Input: part model. Units: mm. Frame: model coordinates. Coordinates: 2 decimals unless noted, no trailing zeros. Write each loop counter-clockwise with the first axis right and the second up, starting at its lowest first coordinate (ties: lowest second). Pieces come first, ordered by that corner, then holes. Notation, with made-up numbers: (-18.75, 47.5) -> (11.25, 47.5) arc R34 cw to (11.25, 81.5) -> close; hole circle Ø4 at (-16.5, 6). An arc over 180 degrees is marked (long way). Use one line per item in the form item = value. Start each with the question number.
(1) Ray query, line 1 along Z through (x, y) = (-4.5, 0); line 2 along Y through (x, z) = (-4.4, 290); line 3 along Y through (x, z) = (-1, 153.5). Return the intervals inside material, ascending.
(2) Cut plane C-C on z = 158. Return the cut outline in (x, y).
(3) First-contact query: pin 1 (1.5 mm diameter, centred on x = 2, y = 0.5, fed in from -Z). Flat tip, straight axial feed; report the tip coordinate or a pass-through.
(4) Cut plane A-A on x = 0. Return the cut outline in (y, z), plus the area to 3 significant figures.
(5) Cut plane B-B on y = 0. Return the cut outline in (x, z).
Autodesk Inventor part; units mm, degrees
ref_plane "YZ Plane" through (0, 0, 0) normal (1, 0, 0) x (0, 1, 0)
ref_plane "XZ Plane" through (0, 0, 0) normal (0, 1, 0) x (-1, 0, 0)
ref_plane "XY Plane" through (0, 0, 0) normal (0, 0, 1) x (1, 0, 0)
sketch "スケッチ1" plane through (0, 0, 0) normal (0, 0, 1) x (1, 0, 0)
  line L0 (5, -5) -> (-5, -5)
  line L1 (-5, -5) -> (-5, 5)
  line L2 (-5, 5) -> (5, 5)
  line L3 (5, 5) -> (5, -5)
  line L4 (5, -5) -> (-5, 5) construction
  line L5 (-5, -5) -> (5, 5) construction
  line L6 (4, 4) -> (-4, 4)
  line L7 (-4, 4) -> (-4, -4)
  line L8 (-4, -4) -> (4, -4)
  line L9 (4, -4) -> (4, 4)
  point P0 (0, 0)
  dimension "d0" = 10
  dimension "d1" = 10
  dimension "d2" = 1
extrude "押し出し1" add sketch "スケッチ1" along normal blind 300
sketch "スケッチ2" plane through (5, -5, 0) normal (1, 0, 0) x (0, 0, -1)
  line L0 (0, 0) -> (0, 10)
  line L1 (0, 10) -> (-300, 10)
  line L2 (-300, 0) -> (-300, 10)
  line L3 (0, 0) -> (-300, 0)
  line L4 (-300, 5) -> (0, 5)
  point P0 (-290, 5)
  point P1 (-10, 5)
  dimension "d5" = 280
  dimension "d7" = 10
hole "穴1" at (5, 0, 290) at (5, 0, 10) direction (-1, 0, 0) diameter 3.3 end through all
sketch "スケッチ3" plane through (-5, 5, 0) normal (0, 1, 0) x (1, 0, 0)
  line L0 (10, 0) -> (0, 0)
  line L1 (0, 0) -> (0, -300)
  line L2 (10, -300) -> (0, -300)
  line L3 (10, 0) -> (10, -300)
  line L4 (5, 0) -> (5, -300)
  point P0 (5, -150)
hole "穴2" at (0, 5, 150) direction (0, -1, 0) diameter 3.3 end through all
properties part number "kaku_1010_300"
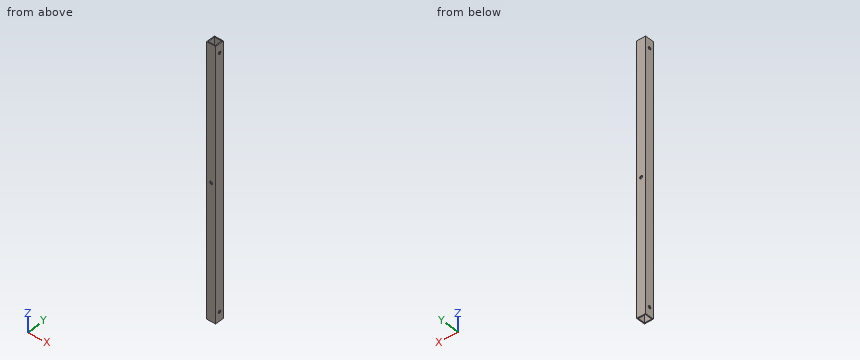
Values:
q1.line_1 = 0 to 8.35, 11.65 to 288.35, 291.65 to 300
q1.line_2 = -5 to -1.65, 1.65 to 5
q1.line_3 = -5 to -4, 4 to 5
q2.outline = (-5, -5) -> (5, -5) -> (5, 5) -> (-5, 5) -> close; hole (-4, -4) -> (4, -4) -> (4, 4) -> (-4, 4) -> close
q3.pin_1 = through
q4.outline = (-5, 0) -> (-4, 0) -> (-4, 148.35) -> (-5, 148.35) -> close; (-5, 151.65) -> (-4, 151.65) -> (-4, 300) -> (-5, 300) -> close; (4, 0) -> (5, 0) -> (5, 148.35) -> (4, 148.35) -> close; (4, 151.65) -> (5, 151.65) -> (5, 300) -> (4, 300) -> close
q4.area = 593 mm2
q5.outline = (-5, 0) -> (-4, 0) -> (-4, 8.35) -> (-5, 8.35) -> close; (-5, 11.65) -> (-4, 11.65) -> (-4, 288.35) -> (-5, 288.35) -> close; (-5, 291.65) -> (-4, 291.65) -> (-4, 300) -> (-5, 300) -> close; (4, 0) -> (5, 0) -> (5, 8.35) -> (4, 8.35) -> close; (4, 11.65) -> (5, 11.65) -> (5, 288.35) -> (4, 288.35) -> close; (4, 291.65) -> (5, 291.65) -> (5, 300) -> (4, 300) -> close
